Can you work these out from the drawing? Everything is in mm from the part's minimum corner. A direction names the side the tool comes from. Round coordinates to 2 decimals unless told otherwise and drop trailing zeros. Write each loop counter-clockwise with the first axis right and the second up, starting at its lowest first coordinate (ties: lowest second). Pieces come first, ordered by that corner, then holes. Notation, with made-up numbers: (74, -5) - (133, -5) arc R21 cw to (133, 27) - close; hole circle Ø10 at (-23.5, -25.5). An arc over 180 degrees is marked (long way). One line per item, written item: value. Start each with the question number.
(1) I want a section at D-D on x = 25. List the corners of the cut face in (y, z) for me, plus the area to 3 significant figures.
(2) On a 3-axis mill with a long thin cutter (end or side, diameter ignored), from which of +Z, -Z, +X, -X, +Y, -Y can I reach the whole of each face in a straight line? I mean the marked faces 4 and 5. Say none if no direction works.
(3) I want a section at A-A on x = 16. List the corners of the cut face in (y, z) for me, plus the area to 3 significant figures.
(4) If I drill on L1, parallel to Y at x = 16, z = 2.85; L2, parallel to X at y = 50, z = 1.95; L3, parallel to X at y = 23.5, z = 3.2, over which ranges is the centre line in solid material (lowest first)? Write a range as from..to.
(5) Thinking about a two-plate mould opening in X: for the marked faces 1, 2 and 3, which applies, +X half, -X half, draft (parallel to the pull), parting line (faces both ways), or undercut?
(6) I want a section at B-B on z = 1.75. List the corners of the cut face in (x, y) for me.
(7) I'm going to push flat-ended pins straight in: pin 1 Ø1.5 at (y, z) = (13.5, 2) entering from +X; pin 2 Ø3 at (x, y) = (27.69, 56.75) entering from +Z; pin 3 Ø3 at (x, z) = (27.5, 4.5) entering from -Y; pin 4 Ø1.5 at (y, z) = (13, 1.5) entering from -X. Where does each tip first touch, or does it pass through?
(8) I want a section at C-C on y = 50. List the corners of the cut face in (x, z) for me, plus the area to 3 significant figures.
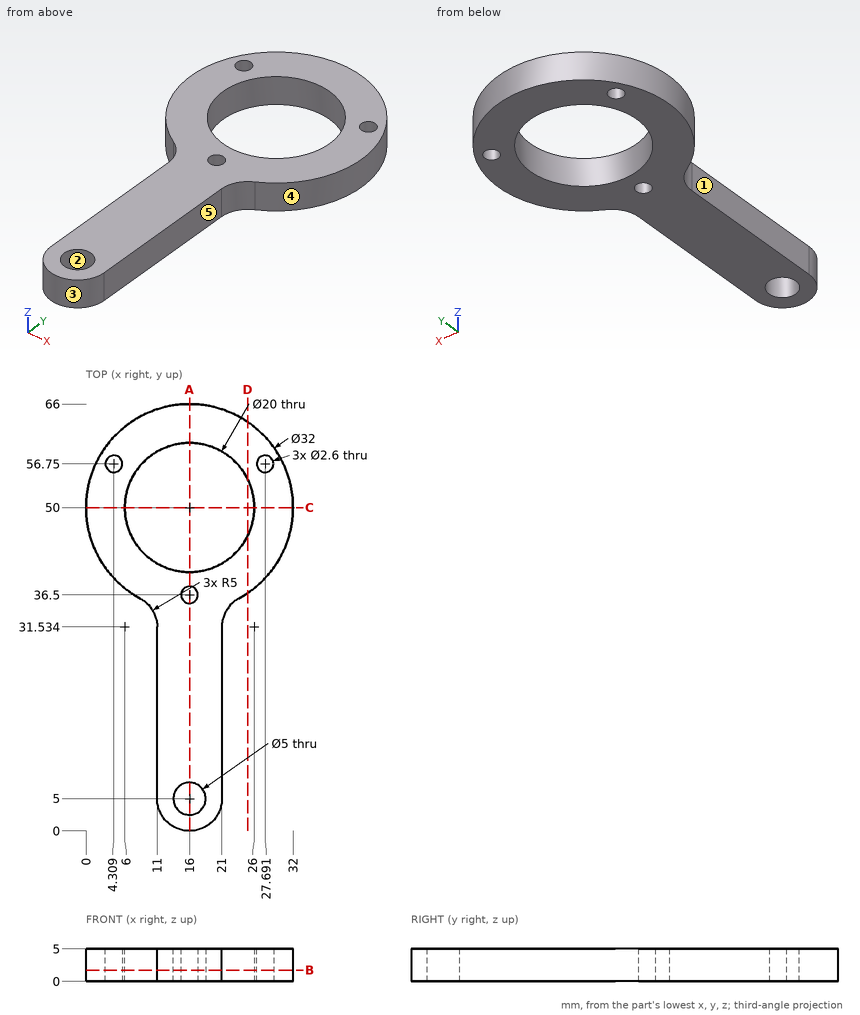
Established:
1. outline: (36.77, 0) - (45.64, 0) - (45.64, 5) - (36.77, 5) - close; (54.36, 0) - (63.23, 0) - (63.23, 5) - (54.36, 5) - close
1. area: 88.7 mm2
2. face 4: +Z, -Z
2. face 5: +Z, -Z, +X, -Y
3. outline: (0, 0) - (2.5, 0) - (2.5, 5) - (0, 5) - close; (7.5, 0) - (35.2, 0) - (35.2, 5) - (7.5, 5) - close; (37.8, 0) - (40, 0) - (40, 5) - (37.8, 5) - close; (60, 0) - (66, 0) - (66, 5) - (60, 5) - close
3. area: 192 mm2
4. L1: 0..2.5, 7.5..35.2, 37.8..40, 60..66
4. L2: 0..6, 26..32
4. L3: 11..21
5. face 1: -X half
5. face 2: undercut
5. face 3: parting line
6. outline: (8.38, 35.93) arc R5 cw to (11, 31.53) - (11, 5) arc R5 ccw to (21, 5) - (21, 31.53) arc R5 cw to (23.62, 35.93) arc R16 ccw (long way) to start; hole circle Ø2.6 at (4.31, 56.75); hole circle Ø20 at (16, 50); hole circle Ø5 at (16, 5); hole circle Ø2.6 at (16, 36.5); hole circle Ø2.6 at (27.69, 56.75)
7. pin 1: x = 21
7. pin 2: z = 5
7. pin 3: y = 37.51
7. pin 4: x = 11
8. outline: (0, 0) - (6, 0) - (6, 5) - (0, 5) - close; (26, 0) - (32, 0) - (32, 5) - (26, 5) - close
8. area: 60.0 mm2
